Job drawing, mm, ordinate dimensions from the low corner. One solid piece. A direction names the side the tool comes from. Round coordinates to 2 decimals unless told otherwise and drop trailing zeros. Loops run counter-clockwise (first coordinate to the right, second up) from the corner with the lowest first, then second, coordinate; pieces in that order, holes last. Notation, with made-up numbers: M 46.5,-39.5 L 99.5,-39.5 A23 cw 99.5,-17.5 Z; hole C 70.25,-18 d8. An arc over 180 degrees is marked long. One line per item, written item: value.
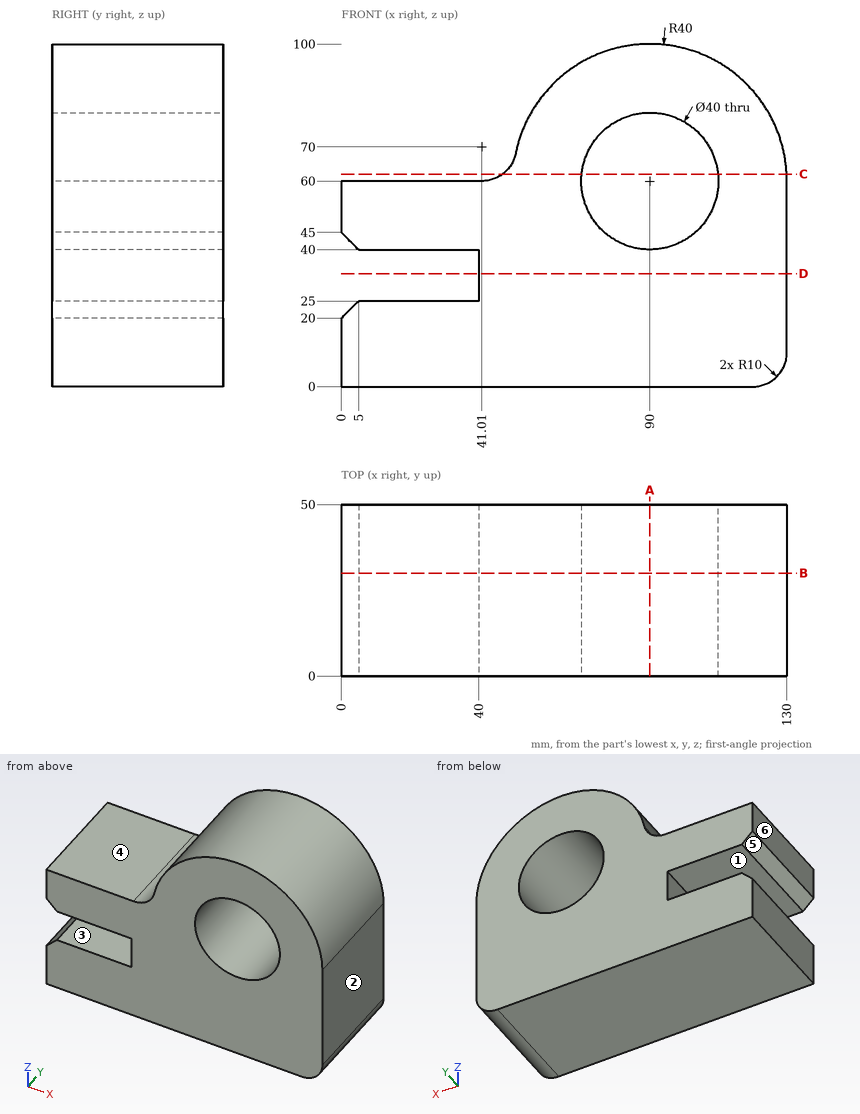
Item 1: Slice it at C-C, the plane z = 62. Give the cut face in (x, y), and give its area (3 significant figures).
Check values:
outline: M 47.01,0 L 70.1,0 L 70.1,50 L 47.01,50 Z; M 109.9,0 L 129.95,0 L 129.95,50 L 109.9,50 Z
area: 2,160 mm2
Item 2: Pull direction Z, two halves, no side cores. Call the marked faces 1, 2, 3 and 4: pulls with the +Z half, pulls with the -Z half, needs draft (parallel to the pull), parting line crosses it, or undercut.
Check values:
face 1: undercut
face 2: needs draft
face 3: undercut
face 4: pulls with the +Z half
Item 3: Slice it at A-A, the plane x = 90. Give the cut face in (y, z).
Check values:
outline: M 0,0 L 50,0 L 50,40 L 0,40 Z; M 0,80 L 50,80 L 50,100 L 0,100 Z
Item 4: Drop flat-ended pins along their axis: P1, Ø1.5, axis at y = 37, z = 15, coming from the -X side; P2, Ø17.5, axis at x = 24.5, y = 36.5, coming from the +Z side; P3, Ø2, axis at x = 111.5, y = 39, coming from the +Z side; P4, Ø3, axis at y = 15, z = 24, coming from the -X side. Give the stop position or say it passes through.
Check values:
P1: stops at x = 0
P2: stops at z = 60
P3: stops at z = 94.35
P4: stops at x = 2.5
Item 5: Wall check: line 1 along Z through (x, y) = (20, 29.5); line 2 along Z through (x, y) = (90, 11); line 3 along X through (y, z) = (23, 74). Give the ranges that are in metal, low to high.
Check values:
line 1: z = 0 to 25, 40 to 60
line 2: z = 0 to 40, 80 to 100
line 3: x = 52.53 to 75.72, 104.28 to 127.47
Item 6: Slice it at B-B, the plane y = 30. Give the cut face in (x, z), and give its area (3 significant figures).
Check values:
outline: M 0,0 L 120,0 A10 ccw 130,10 L 130,60 A40 ccw 50.81,68 A10 cw 41.01,60 L 0,60 L 0,45 L 5,40 L 40,40 L 40,25 L 5,25 L 0,20 Z; hole C 90,60 d40
area: 8,430 mm2
Item 7: Which spindle directions (+Z, -Z, +X, -X, +Y, -Y) get a long thin tool onto all of the face, cutting with end or side? Do the marked faces 5 and 6. Say none if no direction does.
Check values:
face 5: -X, +Y, -Y
face 6: +Z, -Z, -X, +Y, -Y
Item 8: Slice it at D-D, the plane z = 33. Give the cut face in (x, y), and give its area (3 significant figures).
Check values:
outline: M 40,0 L 130,0 L 130,50 L 40,50 Z
area: 4,500 mm2
